```python
from build123d import *

# Parameters (mm, degrees)
RESSALTO_EXTRUS_O1_DEPTH = 90
ESBO_O3_W                = 91
ESBO_O3_H                = 84
ESBO_O4_R                = 1.5
CORTE_EXTRUS_O1_DEPTH    = 113.517776373


with BuildPart() as part:
    # Esboço1 → Ressalto-extrusão1 (new body)
    with BuildSketch(Plane(origin=(0, 0, 0), x_dir=(1, 0, 0), z_dir=(0, 1, 0))):
        with BuildLine():
            Line((0, 0), (64.5, 0))
            Line((64.5, 0), (64.5, 9.312094154))
            ThreePointArc((64.5, 9.312094154), (32.25, 20), (0, 9.312094154))
            Line((0, 9.312094154), (0, 0))
        make_face()
    extrude(amount=RESSALTO_EXTRUS_O1_DEPTH)

    # Esboço3 → Corte-Revolução2 (revolve, cut)
    with BuildSketch(Plane(origin=(32.25, 0, 0), x_dir=(0, 0, -1), z_dir=(1, 0, 0))):
        with Locations((-30.5, 45)):
            Rectangle(ESBO_O3_W, ESBO_O3_H)
    revolve(axis=Axis((32.25, 87, 76), (0, -1, 0)), mode=Mode.SUBTRACT)

    # Esboço4 → Corte-extrusão1 (cut, through all)
    with BuildSketch(Plane(origin=(0, 90, 0), x_dir=(1, 0, 0), z_dir=(0, 1, 0))):
        with Locations(Location((7.24, 5.82, 0), (0, 0, 270))):
            Circle(ESBO_O4_R)
        with Locations(Location((57.26, 5.82, 0), (0, 0, 270))):
            Circle(ESBO_O4_R)
    extrude(amount=-CORTE_EXTRUS_O1_DEPTH, mode=Mode.SUBTRACT)


solid = part.part
```
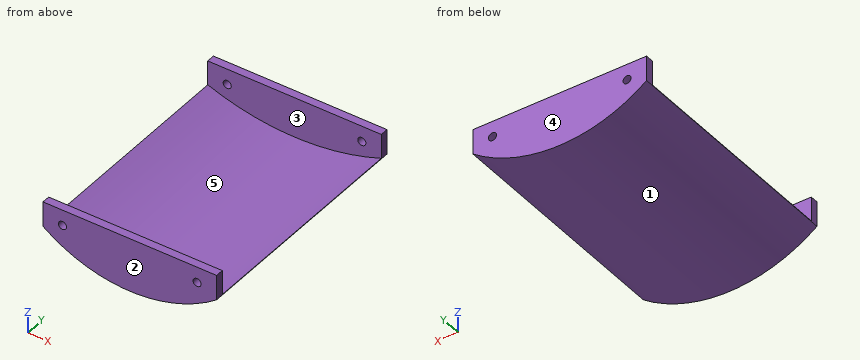
For this review, take the finished solid that the model builds, in its own axes (mm). Face numbers are marked on the shaded views. A direction names the side the tool comes from. Coordinates: 2 decimals unless noted, no trailing zeros. Order: outer loops, then holes, each group sorted by start corner. A loop starts at its lowest first (then second) coordinate and runs counter-clockwise, first axis right, second up. Notation, with made-up numbers: (-39, -17) - (-10, -17) arc R27 ccw to (-10, 15) - close; hole circle Ø4 at (-14, 22). An arc over 180 degrees is marked (long way). Answer as a JSON object with one key per item and string values. Group by question number.
1. The part is to be moulded in two halves that separate along Y. For the marked faces 1, 2 and 3, say which applies: pulls with the +Y half, pulls with the -Y half, needs draft (parallel to the pull), parting line crosses it, or undercut.
2. We need section C-C on z = -12. State the section outline as (x, y) points, then the cut area to 3 significant figures.
3. For probe 1 along X at (y, z) = (88.4, -5.82); probe 2 along Y at (x, z) = (34, -4); probe 3 along Z at (x, y) = (7, 1), list the stretches that pass through material, from the lowest coordinate up.
4. We need section D-D on x = 50. State the section outline as (y, z) points.
5. We need section B-B on x = 57.26. State the section outline as (y, z) points, then the cut area to 3 significant figures.
6. We need section A-A on z = -5.82. State the section outline as (x, y) points, then the cut area to 3 significant figures.
7. For the marked faces 4 and 5, list the 3-axis set-ups (+Z, -Z, +X, -X, +Y, -Y) from which the entire face can be reached by the end or side of a thin tool; tool diameter is ignored.
8. Clearance check with flat-ended pins moving along their axes: P1, Ø3, axis at y = 13.5, z = -11.5, coming from the +X side; P2, Ø5, axis at y = 22, z = -13, coming from the -X side; P3, Ø6, axis at x = 22, y = 54.5, coming from the +Z side. State where each tip first meets the part, or that it passes through.
Final values:
{
 "1": {"face 1": "needs draft", "face 2": "pulls with the -Y half", "face 3": "undercut"},
 "2": {"outline": "(3.97, 0) - (60.53, 0) - (60.53, 90) - (3.97, 90) - close; hole (9.08, 3) - (55.42, 3) - (55.42, 87) - (9.08, 87) - close", "area": "1,200 mm²"},
 "3": {"probe 1": "0 to 5.74, 8.74 to 55.76, 58.76 to 64.5", "probe 2": "0 to 3, 87 to 90", "probe 3": "-13.73 to -7.3, -4.34 to 0"},
 "4": {"outline": "(0, -17) - (90, -17) - (90, 0) - (87, 0) - (87, -13.25) - (3, -13.25) - (3, 0) - (0, 0) - close"},
 "5": {"outline": "(0, -13.86) - (90, -13.86) - (90, -7.32) - (87, -7.32) - (87, -11.5) - (3, -11.5) - (3, -7.32) - (0, -7.32) - close; (0, -4.32) - (3, -4.32) - (3, 0) - (0, 0) - close; (87, -4.32) - (90, -4.32) - (90, 0) - (87, 0) - close", "area": "264 mm²"},
 "6": {"outline": "(0, 0) - (5.74, 0) - (5.74, 3) - (0, 3) - close; (0, 87) - (5.74, 87) - (5.74, 90) - (0, 90) - close; (8.74, 0) - (55.76, 0) - (55.76, 3) - (8.74, 3) - close; (8.74, 87) - (55.76, 87) - (55.76, 90) - (8.74, 90) - close; (58.76, 0) - (64.5, 0) - (64.5, 3) - (58.76, 3) - close; (58.76, 87) - (64.5, 87) - (64.5, 90) - (58.76, 90) - close", "area": "351 mm²"},
 "7": {"face 4": "+Z, -Z, +X, -X, +Y", "face 5": "+Z"},
 "8": {"P1": "x = 63.55", "P2": "x = 1.66", "P3": "z = -14.03"}
}
